```python
from build123d import *

# Parameters (mm, degrees)
F0_W        = 5
F0_H        = 16
F1_DEPTH    = 5
F2_R        = 4.49999
F3_T1_DEPTH = 22.5
F4_R        = 3
F5_R        = 4.5
F6_DEPTH    = 2.5
F7_R        = 2.65
F8_DEPTH    = 25
F9_R        = 7


# Not quite as in the source:
# - a fillet or chamfer that OpenCascade refuses, or shapes differently, is made with other operations: its cross-section is extruded or revolved along the edge and cut away or added
# - a fillet or chamfer is up to 0.001 mm smaller than in the source, because OpenCascade refuses the exact size


with BuildPart() as f1:
    # F0 (on Front) → F1 (new body)
    with BuildSketch(Plane.XZ):
        with BuildLine():
            Line((8.5, 12.5), (2.5, 12.5))
            Line((2.5, 12.5), (2.5, 11.1622776602))
            ThreePointArc((2.5, 11.1622776602), (5.8708286934, 10.9580398915), (7.5, 8))
            ThreePointArc((7.5, 8), (5.8708286934, 5.0419601085), (2.5, 4.8377223398))
            Line((2.5, 4.8377223398), (2.5, 3.5))
            Line((2.5, 3.5), (8.5, 3.5))
            Line((8.5, 3.5), (8.5, 12.5))
        make_face()
        with BuildLine():
            Line((-2.5, 11.1622776602), (-2.5, 12.5))
            Line((-2.5, 12.5), (-8.5, 12.5))
            Line((-8.5, 12.5), (-8.5, 3.5))
            Line((-8.5, 3.5), (-2.5, 3.5))
            Line((-2.5, 3.5), (-2.5, 4.8377223398))
            ThreePointArc((-2.5, 4.8377223398), (-7.5, 8), (-2.5, 11.1622776602))
        make_face()
        with BuildLine():
            Line((2.5, 11.1622776602), (2.5, 12.5))
            Line((2.5, 12.5), (-2.5, 12.5))
            Line((-2.5, 12.5), (-2.5, 11.1622776602))
            ThreePointArc((-2.5, 11.1622776602), (-1.0419601085, 9.8708286934), (-0.5, 8))
            ThreePointArc((-0.5, 8), (-1.0419601085, 6.1291713066), (-2.5, 4.8377223398))
            Line((-2.5, 4.8377223398), (-2.5, 3.5))
            Line((-2.5, 3.5), (2.5, 3.5))
            Line((2.5, 3.5), (2.5, 4.8377223398))
            ThreePointArc((2.5, 4.8377223398), (0.5, 8), (2.5, 11.1622776602))
        make_face()
        with Locations((0, -4.5)):
            Rectangle(F0_W, F0_H)
    extrude(amount=F1_DEPTH)

    # F2 (radius 4.5 in the source; OpenCascade refuses exactly that, so slightly less here)
    f2_edges = [f1.edges().sort_by_distance(p)[0] for p in [
        (8.5, -2.5, 12.5),
        (-8.5, -2.5, 12.5),
        (8.5, -2.5, 3.5),
        (-8.5, -2.5, 3.5),
    ]]
    fillet(f2_edges, radius=F2_R)

    # F3: fillet of radius 3.5 on 2 edges, made by hand

    # F3_s2 → F3_t1 (cut)
    with BuildSketch(Plane.YZ.offset(-11.25)):
        with BuildLine():
            ThreePointArc((0, -9), (-1.0251262658, -11.4748737342), (-3.5, -12.5))
            Line((-3.5, -12.5), (0, -12.5))
            Line((0, -12.5), (0, -9))
        make_face()
        with BuildLine():
            ThreePointArc((-5, -9), (-3.9748737342, -11.4748737342), (-1.5, -12.5))
            Line((-1.5, -12.5), (-5, -12.5))
            Line((-5, -12.5), (-5, -9))
        make_face()
    extrude(amount=F3_T1_DEPTH, mode=Mode.SUBTRACT)

    # F4
    f4_edges = [f1.edges().sort_by_distance(p)[0] for p in [
        (2.5, -2.5, 3.5),
        (-2.5, -2.5, 3.5),
    ]]
    fillet(f4_edges, radius=F4_R)

    # F5 (on Right) → F6 (join, symmetric)
    with BuildSketch(Plane.YZ):
        with Locations((-2.5, -9)):
            Circle(F5_R)
    extrude(amount=F6_DEPTH, both=True)

    # F7 (on face) → F8 (cut)
    with BuildSketch(Plane.YZ.offset(2.5)):
        with Locations((-2.5, -9)):
            Circle(F7_R)
    extrude(amount=-F8_DEPTH, mode=Mode.SUBTRACT)

    # F9
    f9_edges = [f1.edges().sort_by_distance(p)[0] for p in [
        (0, 0, -5.258343),
        (0, -5, -5.258343),
    ]]
    fillet(f9_edges, radius=F9_R)


solid = f1.part
```
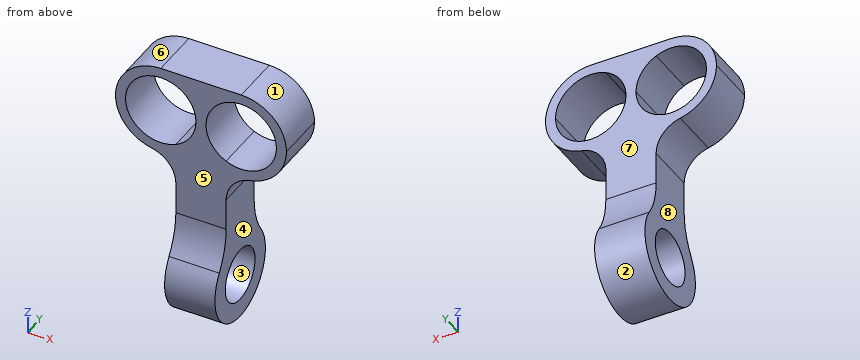
For this review, take the finished solid that the model builds, in its own axes (mm). Face numbers are marked on the shaded views. A direction names the side the tool comes from. Round coordinates to 2 decimals unless told otherwise and drop trailing zeros. Loops run counter-clockwise (first coordinate to the right, second up) from the corner with the lowest first, then second, coordinate; pieces in that order, holes last.
(1) Clearance check with flat-ended pins moving along their axes: P1, Ø4.5, axis at x = -0.5, z = 7.5, coming from the -Y side; P2, Ø3, axis at x = -3.5, y = -5.5, coming from the -Z side; P3, Ø2, axis at y = -3.5, z = -3, coming from the -X side; P4, Ø6, axis at x = 5, z = -10, coming from the -Y side. State where each tip first meets the part, or that it passes through.
Returned:
P1: stops at y = -5
P2: stops at z = -13.09
P3: stops at x = -2.5
P4: stops at y = -7
(2) We need section C-C (x = -5.75). Give the boundary of the cut face in (y, z).
Returned:
outline: (-5, 3.85) - (0, 3.85) - (0, 4.97) - (-5, 4.97) - close; (-5, 11.03) - (0, 11.03) - (0, 12.15) - (-5, 12.15) - close
(3) Mouldability with a two-part tool opening along Z and no side actions: class the marked faces 1, 2 and 3 as released by +Z, released by -Z, zero draft, split by the parting line, or undercut.
Returned:
face 1: released by +Z
face 2: split by the parting line
face 3: undercut
(4) We need section B-B (y = -2.5). State how many separate pieces and enclosed holes the cut face has, plus the area to 3 significant figures.
Returned:
separate pieces: 2
enclosed holes: 2
area: 120 mm2
(5) Wall thickness on line 1 along X through (y, z) = (-2.65, 8); line 2 along Z through (x, y) = (-1.4, -2.5); line 3 along X through (y, z) = (-3.75, 5.25): over which ranges is each line inside the solid? List them lowest first.
Returned:
line 1: x = -8.5 to -7.5, -0.5 to 0.5, 7.5 to 8.5
line 2: z = -13.5 to -11.65, -6.35 to 5.66, 10.34 to 12.5
line 3: x = -7.56 to -6.17, -1.83 to 1.83, 6.17 to 7.56
(6) Tool access review of the marked faces 4, 5, 6, 7 and 8: name each direction out of +Z, -Z, +X, -X, +Y, -Y from which nothing blocks a thin tool from reaching the whole face with its end or side.
Returned:
face 4: -Z, +X, +Y, -Y
face 5: +Z, +X, -X, -Y
face 6: +Z, -X, +Y, -Y
face 7: +Z, +X, -X, +Y
face 8: -Z, -X, +Y, -Y
(7) We need section A-A (z = -9). Give the boundary of the cut face in (x, y), plus the area to 3 significant figures.
Returned:
outline: (-2.5, -7) - (2.5, -7) - (2.5, -5.15) - (-2.5, -5.15) - close; (-2.5, 0.15) - (2.5, 0.15) - (2.5, 2) - (-2.5, 2) - close
area: 18.5 mm2
